```python
from build123d import *
from build123d.topology import SkipClean

# Parameters (mm, degrees)
SKETCH1_R               = 2.625
BOSS_EXTRUDE1_DEPTH     = 18
SKETCH2_W               = 3.75
SKETCH2_H               = 40
BOSS_EXTRUDE2_DEPTH     = 15.5
CUT_EXTRUDE1_DEPTH      = 3.5
CUT_EXTRUDE2_DEPTH      = 4
CUT_EXTRUDE2_DEPTH_BACK = 4
SKETCH4_W               = 26.185074211
SKETCH4_H               = 43.492971865
CUT_EXTRUDE3_DEPTH      = 3.75


with BuildPart() as part:
    # Sketch1 → Boss-Extrude1 (new body)
    with BuildSketch(Plane(origin=(0, 0, 0), x_dir=(0, 0, -1), z_dir=(1, 0, 0))):
        with BuildLine():
            Line((0, 0), (5, 0))
            Line((5, 0), (5, 40))
            Line((5, 40), (0, 40))
            Line((0, 40), (-2.5, 40))
            Line((-2.5, 40), (-15.763202528, 42.911607583))
            ThreePointArc((-15.763202528, 42.911607583), (-22.576511621, 41.311816677), (-25.6, 35))
            Line((-25.6, 35), (-25.6, 20))
            ThreePointArc((-25.6, 20), (-24.659331675, 16.211336651), (-22.055809883, 13.302642588))
            Line((-22.055809883, 13.302642588), (-2.5, 0))
            Line((-2.5, 0), (0, 0))
        make_face()
        with Locations((-17.5, 35)):
            Circle(SKETCH1_R, mode=Mode.SUBTRACT)
        with Locations((-17.5, 20)):
            Circle(SKETCH1_R, mode=Mode.SUBTRACT)
    extrude(amount=BOSS_EXTRUDE1_DEPTH)

    # Sketch2 → Boss-Extrude2 (add)
    with BuildSketch(Plane.ZY):
        with Locations((-3.125, 20)):
            Rectangle(SKETCH2_W, SKETCH2_H)
    extrude(amount=BOSS_EXTRUDE2_DEPTH)

    # Sketch3 → Cut-Extrude1 (cut)
    with BuildSketch(Plane(origin=(18, 0, 0), x_dir=(0, 0, -1), z_dir=(1, 0, 0))):
        Polygon((-12.881197846, 35), (-15.190598923, 39), (-19.809401077, 39), (-22.118802154, 35), (-19.809401077, 31), (-15.190598923, 31), align=None)
        Polygon((-12.881197846, 20), (-15.190598923, 24), (-19.809401077, 24), (-22.118802154, 20), (-19.809401077, 16), (-15.190598923, 16), align=None)
    cut_extrude1 = extrude(amount=-CUT_EXTRUDE1_DEPTH, mode=Mode.SUBTRACT)

    # Mirror1: Cut-Extrude1 across plane
    add(cut_extrude1.mirror(Plane(origin=(9, 0, 0), x_dir=(0, 0, 1), z_dir=(1, 0, 0))), mode=Mode.SUBTRACT)

    # Sketch4 → Cut-Extrude2 (cut, two sides: drawn at the far end of the back side and taken through both)
    with BuildSketch(Plane(origin=(9, 0, 0), x_dir=(0, 0, -1), z_dir=(1, 0, 0)).offset(-CUT_EXTRUDE2_DEPTH_BACK)):
        with Locations((-19.842537105, 21.746485933)):
            Rectangle(SKETCH4_W, SKETCH4_H)
    extrude(amount=CUT_EXTRUDE2_DEPTH + CUT_EXTRUDE2_DEPTH_BACK, mode=Mode.SUBTRACT)

    # Sketch5 → Cut-Extrude3 (cut)
    with BuildSketch(Plane.XY.offset(-1.25)):
        with BuildLine():
            Line((-15.5, 23.302), (-15.5, 16.698))
            ThreePointArc((-15.5, 16.698), (-12.198, 20), (-15.5, 23.302))
        make_face()
    extrude(amount=-CUT_EXTRUDE3_DEPTH, mode=Mode.SUBTRACT)

    # Mirror2: part across plane


with BuildPart() as part_1:
    with SkipClean():  # the faces are left unmerged after this step: merging them gives an invalid solid
        add(part.part)
        add(part.part.mirror(Plane(origin=(-15.5, 0, 0), x_dir=(0, 0, 1), z_dir=(1, 0, 0))))


solid = part_1.part
```
For this review, take the finished solid that the model builds, in its own axes (mm). A direction names the side the tool comes from. Give positions to 0.01 mm unless a question says otherwise; leave off trailing zeros. Write each loop counter-clockwise with the first axis right and the second up, starting at its lowest first coordinate (ties: lowest second). Pieces come first, ordered by that corner, then holes. Notation, with made-up numbers: M 21.5,31 L 41.5,31 A17 cw 41.5,45 Z; hole C 8,-6.75 d3. An arc over 180 degrees is marked long. Answer as a JSON object with one key per item and string values. Group by question number.
Item 1: For pin 1 Ø1 at (x, z) = (2.5, 18) entering from +Y; pin 2 Ø15.5 at (x, y) = (-9.5, 23.5) entering from +Z; pin 3 Ø1 at (x, z) = (-33, 17) entering from -Y; pin 4 Ø1 at (x, z) = (16, 16.5) entering from -Y, all flat-tipped, find the tip position at first contact; note any pin that passes through.
Item 2: Consider section A-A on x = -15.5. Write out the cut boundary in (y, z).
Item 3: Draft analysis for pull direction Y (two halves, no side actions). For faces 6 (the flat face through (-40, 22, 6.75)), 7 (the flat face through (-33.874, 5.266, 10.242)), 8 (the flat face through (1.73, 18.03, 20.98)), state which applies: +Y half, -Y half, draft (parallel to the pull), parting line (faces both ways), or undercut.
Item 4: Consider section D-D on x = 2.5. Write out the cut boundary in (y, z).
Item 5: Consider section C-C on z = 5.5. Write out the cut boundary in (x, y).
Item 6: Consider section B-B on y = 28. Write out the cut boundary in (x, z).
Item 7: For probe 1 along X at (y, z) = (21, 11); probe 2 along X at (y, z) = (3, 5.5); probe 3 along Z at (x, y) = (-44.5, 35) (3 decimals), list the stretches that pass through material, from the lowest coordinate up. Write a range as [from, to].
Item 8: Tool access review of faces 1 (the flat face through (2, 31, 18)), 2 (the flat face through (-47.274, 22.028, 20.948)), 3 (the flat face through (16.27, 36.97, 14.02)), 4 (the flat face through (-36, 28, 16)), 5 (the flat face through (2, 28, 25.6)): name each direction out of +Z, -Z, +X, -X, +Y, -Y from which nothing blocks a thin tool from reaching the whole face with its end or side.
Check result:
{
 "1": {"pin 1": "stops at y = 43.1", "pin 2": "stops at z = -1.25", "pin 3": "stops at y = 9.52", "pin 4": "stops at y = 9.18"},
 "2": {"outline": "M 0,-5 L 16.7,-5 L 16.7,-1.25 L 0,-1.25 Z; M 23.3,-5 L 40,-5 L 40,-1.25 L 23.3,-1.25 Z"},
 "3": {"face 6": "draft", "face 7": "-Y half", "face 8": "undercut"},
 "4": {"outline": "M 0,-5 L 40,-5 L 40,2.5 L 42.91,15.76 A8.1 ccw 35,25.6 L 20,25.6 A8.1 ccw 13.3,22.06 L 0,2.5 Z; hole M 16,15.19 L 20,12.88 L 24,15.19 L 24,19.81 L 20,22.12 L 16,19.81 Z; hole M 31,15.19 L 35,12.88 L 39,15.19 L 39,19.81 L 35,22.12 L 31,19.81 Z"},
 "5": {"outline": "M -49,2.04 L -31,2.04 L -31,40.66 L -49,40.66 Z; M 0,2.04 L 18,2.04 L 18,40.66 L 0,40.66 Z"},
 "6": {"outline": "M -49,-5 L 18,-5 L 18,25.6 L 13,25.6 L 13,6.75 L 5,6.75 L 5,25.6 L 0,25.6 L 0,-1.25 L -31,-1.25 L -31,25.6 L -36,25.6 L -36,6.75 L -44,6.75 L -44,25.6 L -49,25.6 Z"},
 "7": {"probe 1": "x = [-49, -44], [-36, -31], [0, 5], [13, 18]", "probe 2": "x = [-49, -31], [0, 18]", "probe 3": "z = [-5, 14.875], [20.125, 25.6]"},
 "8": {"face 1": "none", "face 2": "-X", "face 3": "+X", "face 4": "+Z, +Y, -Y", "face 5": "+Z, +X, -X, +Y, -Y"}
}
